Part model, mm, in its own coordinate system. A direction names the side the tool comes from. Round coordinates to 2 decimals unless told otherwise and drop trailing zeros. Order: outer loops, then holes, each group sorted by start corner. A loop starts at its lowest first (then second) coordinate and runs counter-clockwise, first axis right, second up. Notation, with made-up numbers: M 58.5,18.25 L 88.5,18.25 A13 ccw 88.5,32.25 Z; hole C 58,-9.5 d3. An arc over 180 degrees is marked long. Write each question's results on one line, items separated by ' | '. Start each with the question number.
1. Two-plate mould, pull along Y, no slides. Class faces 1 (the face through (65.928, -42.682, 5.423)), 2 (the face through (-15.5, -77, 5)), 3 (the face through (-132.033, -25.391, 5.423)), 4 (the face through (1, -7, 0)): +Y half, -Y half, draft (parallel to the pull), parting line (faces both ways), or undercut.
2. Probe L1, parallel to Y at x = -108, z = 7.75; L2, parallel to Y at x = 15, z = 8.75; L3, parallel to Y at x = 9, z = 2. List the from-to ranges inside material, lowest first. Write a range as [from, to].
3. Band-saw the part on C-C, the plane x = -37. List the corners of the cut face in (y, z).
4. Drop flat-ended pins along their axis: pin 1 Ø4 at (x, z) = (-99, 7.5) entering from -Y; pin 2 Ø1.5 at (y, z) = (-64.5, 3.5) entering from -X; pin 3 Ø4 at (y, z) = (64, 2) entering from -X. Give the stop position or say it passes through.
5. Which spindle directions (+Z, -Z, +X, -X, +Y, -Y) get a long thin tool onto all of the face, cutting with end or side? Do faces 5 (the face through (89.785, 52.953, 5.423)), 6 (the face through (9.5, 123, 5)), 7 (the face through (93.636, -45.362, 5.423)). Say none if no direction does.
6. Band-saw the part on B-B, the plane z = 6.25. Give the number of separate pieces and of enclosed holes in the cut face, then the cut area to 3 significant figures.
7. Band-saw the part on A-A, the plane x = 22.5. List the corners of the cut face in (y, z).
```python
from build123d import *

# Parameters (mm, degrees)
ESQUISSE1_R        = 2
ESQUISSE1_R_2      = 4
ESQUISSE1_R_3      = 2.25
BOSS_EXTRU_1_DEPTH = 11


with BuildPart() as part:
    # Esquisse1 → Boss.-Extru.1 (new body)
    with BuildSketch(Plane.XY):
        with BuildLine():
            Line((55.7582898, 111.889394822), (124.778203229, -7.656601971))
            Line((124.778203229, -7.656601971), (137.475849877, -45.428957942))
            Line((137.475849877, -45.428957942), (128.262549161, -61.386862887))
            Line((128.262549161, -61.386862887), (95.353583818, -42.386862887))
            Line((95.353583818, -42.386862887), (91.869237886, -48.42192707))
            Line((91.869237886, -48.42192707), (48.59232335, -23.435988813))
            ThreePointArc((48.59232335, -23.435988813), (43.128221735, -24.900090428), (44.59232335, -30.364192044))
            Line((44.59232335, -30.364192044), (87.869237886, -55.350130301))
            Line((87.869237886, -55.350130301), (84.941034656, -60.42192707))
            Line((84.941034656, -60.42192707), (117.85, -79.42192707))
            Line((117.85, -79.42192707), (106.4683565, -99.135511886))
            Line((106.4683565, -99.135511886), (69.01991343, -104.23279285))
            Line((69.01991343, -104.23279285), (-69.019913428, -104.23279285))
            Line((-69.019913428, -104.23279285), (-108.080556584, -96.343099429))
            Line((-108.080556584, -96.343099429), (-117.340438531, -80.304513424))
            Line((-117.340438531, -80.304513424), (-84.574106641, -61.386862887))
            Line((-84.574106641, -61.386862887), (-88.01187134, -55.432479764))
            Line((-88.01187134, -55.432479764), (-44.59232335, -30.364192044))
            ThreePointArc((-44.59232335, -30.364192044), (-43.128221735, -24.900090428), (-48.59232335, -23.435988813))
            Line((-48.59232335, -23.435988813), (-92.01187134, -48.504276533))
            Line((-92.01187134, -48.504276533), (-95.205458711, -42.972820948))
            Line((-95.205458711, -42.972820948), (-127.971790601, -61.890471485))
            Line((-127.971790601, -61.890471485), (-139.088049961, -42.636545485))
            Line((-139.088049961, -42.636545485), (-124.77820323, -7.656601972))
            Line((-124.77820323, -7.656601972), (-55.758289801, 111.889394821))
            Line((-55.758289801, 111.889394821), (-29.395293293, 141.772057371))
            Line((-29.395293293, 141.772057371), (-9.5, 141.772057371))
            Line((-9.5, 141.772057371), (-9.5, 103.772057371))
            Line((-9.5, 103.772057371), (-4, 103.772057371))
            Line((-4, 103.772057371), (-4, 53.800180857))
            ThreePointArc((-4, 53.800180857), (0, 49.800180857), (4, 53.800180857))
            Line((4, 53.800180857), (4, 103.772057371))
            Line((4, 103.772057371), (9.5, 103.772057371))
            Line((9.5, 103.772057371), (9.5, 141.772057371))
            Line((9.5, 141.772057371), (32.619693461, 141.772057371))
            Line((32.619693461, 141.772057371), (55.7582898, 111.889394822))
        make_face()
        with Locations((-92.197441117, -35.909709372)):
            Circle(ESQUISSE1_R, mode=Mode.SUBTRACT)
        with Locations((-66.216679003, -20.909709372)):
            Circle(ESQUISSE1_R, mode=Mode.SUBTRACT)
        with Locations((-51.216679003, -46.890471485)):
            Circle(ESQUISSE1_R, mode=Mode.SUBTRACT)
        with Locations((-77.197441117, -61.890471485)):
            Circle(ESQUISSE1_R, mode=Mode.SUBTRACT)
        with Locations((-15, 97.800180857)):
            Circle(ESQUISSE1_R, mode=Mode.SUBTRACT)
        with Locations((-15, 67.800180857)):
            Circle(ESQUISSE1_R, mode=Mode.SUBTRACT)
        with Locations((15, 67.800180857)):
            Circle(ESQUISSE1_R, mode=Mode.SUBTRACT)
        with Locations((15, 97.800180857)):
            Circle(ESQUISSE1_R, mode=Mode.SUBTRACT)
        with Locations((22.5, 119.800180857)):
            Circle(ESQUISSE1_R_2, mode=Mode.SUBTRACT)
        with Locations((-22.5, 119.800180857)):
            Circle(ESQUISSE1_R_2, mode=Mode.SUBTRACT)
        with Locations((-115, -40.414518843)):
            Circle(ESQUISSE1_R_2, mode=Mode.SUBTRACT)
        with Locations((-92.5, -79.385662014)):
            Circle(ESQUISSE1_R_2, mode=Mode.SUBTRACT)
        with Locations((92.5, -79.385662014)):
            Circle(ESQUISSE1_R_2, mode=Mode.SUBTRACT)
        with Locations((115, -40.414518843)):
            Circle(ESQUISSE1_R_2, mode=Mode.SUBTRACT)
        with Locations((92.197441117, -35.909709372)):
            Circle(ESQUISSE1_R, mode=Mode.SUBTRACT)
        with Locations((66.216679003, -20.909709372)):
            Circle(ESQUISSE1_R, mode=Mode.SUBTRACT)
        with Locations((51.216679003, -46.890471485)):
            Circle(ESQUISSE1_R, mode=Mode.SUBTRACT)
        with Locations((77.197441117, -61.890471485)):
            Circle(ESQUISSE1_R, mode=Mode.SUBTRACT)
        with Locations((0, -74.885662014)):
            Circle(ESQUISSE1_R_2, mode=Mode.SUBTRACT)
        with Locations((-76.25, -79.385662014)):
            Circle(ESQUISSE1_R_3, mode=Mode.SUBTRACT)
        with Locations((-108.75, -79.385662014)):
            Circle(ESQUISSE1_R_3, mode=Mode.SUBTRACT)
        with Locations(Location((-106.875, -26.341606032, 0), (0, 0, 180))):
            Circle(ESQUISSE1_R_3, mode=Mode.SUBTRACT)
        with Locations(Location((-123.125, -54.487431655, 0), (0, 0, 180))):
            Circle(ESQUISSE1_R_3, mode=Mode.SUBTRACT)
        with Locations(Location((14.375, 133.873093668, 0), (0, 0, 180))):
            Circle(ESQUISSE1_R_3, mode=Mode.SUBTRACT)
        with Locations(Location((30.625, 105.727268045, 0), (0, 0, 180))):
            Circle(ESQUISSE1_R_3, mode=Mode.SUBTRACT)
        with Locations((-14.375, 133.873093668)):
            Circle(ESQUISSE1_R_3, mode=Mode.SUBTRACT)
        with Locations((-30.625, 105.727268045)):
            Circle(ESQUISSE1_R_3, mode=Mode.SUBTRACT)
        with Locations(Location((108.75, -79.385662014, 0), (0, 0, 180))):
            Circle(ESQUISSE1_R_3, mode=Mode.SUBTRACT)
        with Locations(Location((76.25, -79.385662014, 0), (0, 0, 180))):
            Circle(ESQUISSE1_R_3, mode=Mode.SUBTRACT)
        with Locations((123.125, -54.487431655)):
            Circle(ESQUISSE1_R_3, mode=Mode.SUBTRACT)
        with Locations((106.875, -26.341606032)):
            Circle(ESQUISSE1_R_3, mode=Mode.SUBTRACT)
        with BuildLine():
            Line((-15.5, -67.285662014), (-15.5, -86.485662014))
            ThreePointArc((-15.5, -86.485662014), (-18.9, -89.885662014), (-22.3, -86.485662014))
            Line((-22.3, -86.485662014), (-22.3, -67.285662014))
            ThreePointArc((-22.3, -67.285662014), (-18.9, -63.885662014), (-15.5, -67.285662014))
        make_face(mode=Mode.SUBTRACT)
        with BuildLine():
            Line((12.7, -67.285662014), (12.7, -71.485662014))
            ThreePointArc((12.7, -71.485662014), (9.3, -74.885662014), (5.9, -71.485662014))
            Line((5.9, -71.485662014), (5.9, -67.285662014))
            ThreePointArc((5.9, -67.285662014), (9.3, -63.885662014), (12.7, -67.285662014))
        make_face(mode=Mode.SUBTRACT)
    extrude(amount=BOSS_EXTRU_1_DEPTH)


solid = part.part
```
Solution:
1) face 1: undercut | face 2: undercut | face 3: +Y half | face 4: draft
2) L1: [-96.36, -81.51], [-77.26, -74.91], [-50.36, -28.29], [-24.39, 21.4] | L2: [-104.23, 65.8], [69.8, 95.8], [99.8, 131.71], [136.03, 141.77] | L3: [-104.23, -74.87], [-63.9, 103.77]
3) outline: M -104.23,0 L 133.15,0 L 133.15,11 L -104.23,11 Z
4) pin 1: y = -98.58 | pin 2: x = -91.27 | pin 3: x = -84.56
5) face 5: +Z, -Z, +X, +Y | face 6: +Z, -Z, +Y | face 7: +Z, -Z
6) separate pieces: 1 | enclosed holes: 33 | area: 43,600 mm^2
7) outline: M -104.23,0 L 115.8,0 L 115.8,11 L -104.23,11 Z; M 123.8,0 L 141.77,0 L 141.77,11 L 123.8,11 Z
